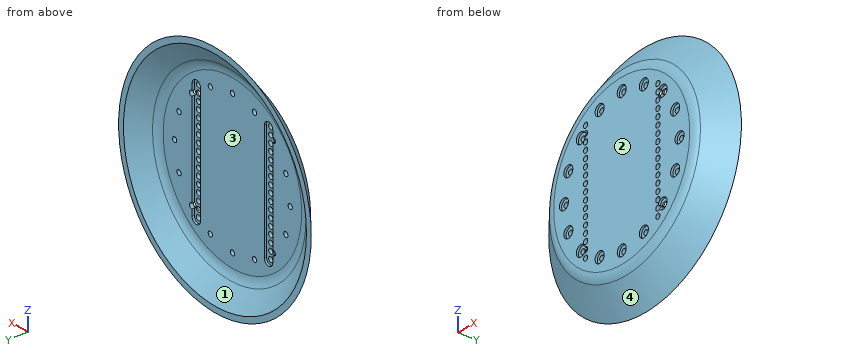
from build123d import *

# Parameters (mm, degrees)
SKETCH2_R            = 1.75
CUT_EXTRUDE1_DEPTH   = 17
LPATTERN1_COUNT      = 9
LPATTERN1_PITCH      = 5
LPATTERN1_COUNT_DIR2 = 5
LPATTERN1_PITCH_DIR2 = 10
SKETCH3_R            = 1.75
CUT_EXTRUDE2_DEPTH   = 17
SKETCH4_R            = 3.75
CUT_EXTRUDE3_DEPTH   = 1.5
CIRPATTERN1_COUNT    = 16
CUT_EXTRUDE4_DEPTH   = 1.5


with BuildPart() as part:
    # Sketch1 → Revolve1 (revolve)
    with BuildSketch(Plane.XY):
        with BuildLine():
            Line((0, 0), (-56.492189406, 0))
            ThreePointArc((-56.492189406, 0), (-59.802258821, 0.563716808), (-62.739139882, 2.191311906))
            Line((-62.739139882, 2.191311906), (-80, 16))
            Line((-80, 16), (-75.998047352, 16))
            Line((-75.998047352, 16), (-63.737187234, 6.191311906))
            ThreePointArc((-63.737187234, 6.191311906), (-60.800306172, 4.563716808), (-57.490236758, 4))
            Line((-57.490236758, 4), (0, 4))
            Line((0, 4), (0, 0))
        make_face()
    revolve(axis=Axis((0, 4, 0), (0, -1, 0)))

    # Sketch2 → Cut-Extrude1 (cut, through all)
    with BuildSketch(Plane.XZ):
        with Locations((-30, 0)):
            Circle(SKETCH2_R)
        with Locations((30, 0)):
            Circle(SKETCH2_R)
    cut_extrude1 = extrude(amount=-CUT_EXTRUDE1_DEPTH, mode=Mode.SUBTRACT)

    # LPattern1: Cut-Extrude1 9 × 5
    with Locations(*[Vector(0, 0, 1) * (i * LPATTERN1_PITCH) + Vector(0, 0, -1) * (j * LPATTERN1_PITCH_DIR2) for i in range(LPATTERN1_COUNT) for j in range(LPATTERN1_COUNT_DIR2) if (i, j) != (0, 0)]):
        add(cut_extrude1, mode=Mode.SUBTRACT)

    # Sketch3 → Cut-Extrude2 (cut, through all)
    with BuildSketch(Plane.XZ):
        with Locations((0, 48)):
            Circle(SKETCH3_R)
    cut_extrude2 = extrude(amount=-CUT_EXTRUDE2_DEPTH, mode=Mode.SUBTRACT)

    # Sketch4 → Cut-Extrude3 (cut)
    with BuildSketch(Plane.XZ):
        with Locations((0, 48)):
            Circle(SKETCH4_R)
    cut_extrude3 = extrude(amount=-CUT_EXTRUDE3_DEPTH, mode=Mode.SUBTRACT)

    # CirPattern1: Cut-Extrude2, Cut-Extrude3 ×16 about axis
    cirpattern1_axis = Axis((0, 0, 0), (0, 1, 0))
    for i in range(1, CIRPATTERN1_COUNT):
        add(cut_extrude2.rotate(cirpattern1_axis, i * 360 / CIRPATTERN1_COUNT), mode=Mode.SUBTRACT)
        add(cut_extrude3.rotate(cirpattern1_axis, i * 360 / CIRPATTERN1_COUNT), mode=Mode.SUBTRACT)

    # Sketch5 → Cut-Extrude4 (cut)
    with BuildSketch(Plane(origin=(0, 4, 0), x_dir=(1, 0, 0), z_dir=(0, 1, 0))):
        with BuildLine():
            Line((-26.5, 40), (-26.5, -40))
            ThreePointArc((-26.5, -40), (-30, -43.5), (-33.5, -40))
            Line((-33.5, -40), (-33.5, 40))
            ThreePointArc((-33.5, 40), (-30, 43.5), (-26.5, 40))
        make_face()
        with BuildLine():
            Line((33.5, 40), (33.5, -40))
            ThreePointArc((33.5, -40), (30, -43.5), (26.5, -40))
            Line((26.5, -40), (26.5, 40))
            ThreePointArc((26.5, 40), (30, 43.5), (33.5, 40))
        make_face()
    extrude(amount=-CUT_EXTRUDE4_DEPTH, mode=Mode.SUBTRACT)


solid = part.part
Can you work these out from the model? Positions are in its coordinate system, mm. Face numbers are marked on the shaded views. Round coordinates to 2 decimals unless told otherwise and drop trailing zeros. Write each loop counter-clockwise with the first axis right and the second up, starting at its lowest first coordinate (ties: lowest second). Pieces come first, ordered by that corner, then holes. Notation, with made-up numbers: M 72.25,8 L 125.25,8 A5 cw 125.25,15 Z; hole C 23.25,37 d5. An arc over 180 degrees is marked long. Use a Markdown table: item, result.
Item 1: We'd pull the mould along Z, two halves only. Please class the marked faces 1, 2, 3 and 4: released by +Z, released by -Z, zero draft, split by the parting line, or undercut.
Found:
| item | result |
|---|---|
| face 1 | undercut |
| face 2 | zero draft |
| face 3 | undercut |
| face 4 | split by the parting line |
Item 2: I want a section at A-A (y = 11.5). List the corners of the cut face in (x, z) for me (3 decimals), and give its area (3 significant figures).
Found:
| item | result |
|---|---|
| outline | C 0,0 d148.75; hole C 0,0 d140.746 |
| area | 1,820 mm2 |
Item 3: If I drill on line 1 along X through (y, z) = (2, -48); line 2 along X through (y, z) = (1.25, -29); line 3 along X through (y, z) = (13.25, 8), over which ranges is the centre line in solid material (lowest first)? Write a range as [from, to].
Found:
| item | result |
|---|---|
| line 1 | x = [-40.02, -1.75], [1.75, 40.02] |
| line 2 | x = [-54.04, -31.44], [-28.56, 28.56], [31.44, 54.04] |
| line 3 | x = [-76.14, -72.12], [72.12, 76.14] |
Item 4: For pin 1 Ø3 at (x, z) = (30, 40) entering from +Y; pin 2 Ø5 at (y, z) = (7.5, 17.5) entering from +X; pin 3 Ø3 at (y, z) = (12.5, 55.5) entering from -X; pin 4 Ø2 at (x, z) = (49, -0.5) entering from -Y, each with a flat end and sliding along its axis, tell me the tip position at first contact or that it passes through.
Found:
| item | result |
|---|---|
| pin 1 | passes through |
| pin 2 | stops at x = 70.41 |
| pin 3 | stops at x = -54.5 |
| pin 4 | stops at y = 1.5 |
